Verification items for the finished model (mm, model axes). Round coordinates to 2 decimals unless told otherwise and drop trailing zeros. Write each loop counter-clockwise with the first axis right and the second up, starting at its lowest first coordinate (ties: lowest second). Pieces come first, ordered by that corner, then holes. Notation, with made-up numbers: (65, 54) - (97, 54) arc R15 cw to (97, 67) - close; hole circle Ø8 at (-2.75, -20.75). An arc over 180 degrees is marked (long way). Answer as a JSON object with one key per item and string values. Group by question number.
1) Go/stop test with flat-tipped pins: pin 1 Ø8 at (x, y) = (0, 0) entering from -Z (3 decimals); pin 2 Ø1.5 at (x, z) = (374, -8) entering from +Y; pin 3 Ø3 at (y, z) = (-302.5, -4) entering from +X. Record where each tip stops, or that it passes through.
2) Section check B-B (x = -69). Enter the section's corners in (y, z).
3) Thickness scan on line 1 (Y direction, x = -3, z = -4.5); line 2 (Z direction, x = -96.5, y = -358); line 3 (Y direction, x = 9, z = -8). Record the ranges inside material, lowest first.
4) Section check A-A (y = -445.5). Enter the section's corners in (x, z).
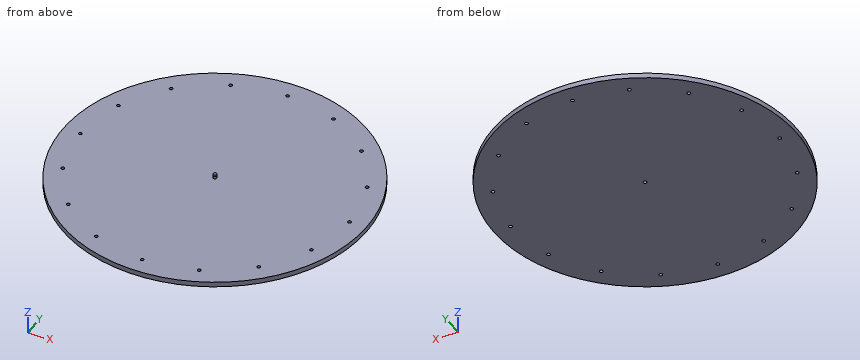
```python
from build123d import *

# Parameters (mm, degrees)
F0_R     = 571.5
F0_R_2   = 6.35
F0_R_3   = 6.604
F1_DEPTH = 19.05
F2_DEPTH = 9.525
F3_DEPTH = 6.35


with BuildPart() as f1:
    # F0 (on Top) → F1 (new body)
    with BuildSketch(Plane.XY):
        Circle(F0_R)
        with Locations((-359.2102448428, -359.2102448428)):
            Circle(F0_R_2, mode=Mode.SUBTRACT)
        with Locations((-194.4031836415, -469.3308025157)):
            Circle(F0_R_2, mode=Mode.SUBTRACT)
        with Locations((-469.3308025157, -194.4031836415)):
            Circle(F0_R_2, mode=Mode.SUBTRACT)
        with Locations((0, -508)):
            Circle(F0_R_2, mode=Mode.SUBTRACT)
        with Locations((194.4031836415, -469.3308025157)):
            Circle(F0_R_2, mode=Mode.SUBTRACT)
        with Locations((359.2102448428, -359.2102448428)):
            Circle(F0_R_2, mode=Mode.SUBTRACT)
        with Locations((469.3308025157, -194.4031836415)):
            Circle(F0_R_2, mode=Mode.SUBTRACT)
        with Locations((-508, 0)):
            Circle(F0_R_2, mode=Mode.SUBTRACT)
        with Locations((-469.3308025157, 194.4031836415)):
            Circle(F0_R_2, mode=Mode.SUBTRACT)
        with Locations((-359.2102448428, 359.2102448428)):
            Circle(F0_R_2, mode=Mode.SUBTRACT)
        with Locations((-194.4031836415, 469.3308025157)):
            Circle(F0_R_2, mode=Mode.SUBTRACT)
        Circle(F0_R_3, mode=Mode.SUBTRACT)
        with Locations((508, 0)):
            Circle(F0_R_2, mode=Mode.SUBTRACT)
        with Locations((469.3308025157, 194.4031836415)):
            Circle(F0_R_2, mode=Mode.SUBTRACT)
        with Locations((0, 508)):
            Circle(F0_R_2, mode=Mode.SUBTRACT)
        with Locations((194.4031836415, 469.3308025157)):
            Circle(F0_R_2, mode=Mode.SUBTRACT)
        with Locations((359.2102448428, 359.2102448428)):
            Circle(F0_R_2, mode=Mode.SUBTRACT)
    extrude(amount=-F1_DEPTH)

    # F0 (on Top) → F2 (join, symmetric)
    with BuildSketch(Plane.XY):
        Circle(F0_R_3)
    extrude(amount=F2_DEPTH, both=True)

    # F3 (add): a face of the model
    f3_faces = [f1.faces().sort_by_distance(p)[0] for p in [
        (0, 0, 9.525),
    ]]
    extrude(f3_faces, amount=F3_DEPTH)


solid = f1.part
```
Returned:
{
 "1": {"pin 1": "z = -9.525", "pin 2": "y = 432.78", "pin 3": "x = 485.81"},
 "2": {"outline": "(-567.32, -19.05) - (567.32, -19.05) - (567.32, 0) - (-567.32, 0) - close"},
 "3": {"line 1": "-571.49 to -513.6, -502.4 to 502.4, 513.6 to 571.49", "line 2": "-19.05 to 0", "line 3": "-571.43 to 571.43"},
 "4": {"outline": "(-357.97, -19.05) - (357.97, -19.05) - (357.97, 0) - (-357.97, 0) - close"}
}
